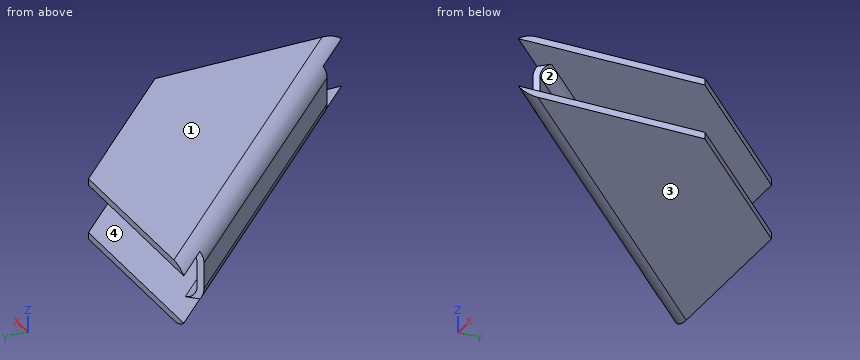
```python
from build123d import *

# Parameters (mm, degrees)
BOSS_EXTRUDE1_START = 6.35
BOSS_EXTRUDE1_DEPTH = 0.762
BOSS_EXTRUDE2_DEPTH = 12.7
FILLET1_R           = 2.54
FILLET2_R           = 4.064


with BuildPart() as part:
    # Sketch4 → Boss-Extrude1 (new, symmetric)
    with BuildSketch(Plane.XY.offset(BOSS_EXTRUDE1_START)):
        Polygon((86.76732538935741, 78.2227633784087), (131.2173253893574, 78.2227633784087), (162.78478969827367, 46.65529906949232), (162.78478969827367, 2.205299069492165), align=None)
    boss_extrude1 = extrude(amount=BOSS_EXTRUDE1_DEPTH, both=True)

    # Sketch5 → Boss-Extrude2 (add)
    with BuildSketch(Plane(origin=(0, 0, 5.588), x_dir=(-1, 0, 0), z_dir=(0, 0, -1))):
        Polygon((-153.41145680361603, 11.578631964150068), (-95.03979201666652, 69.95029675109956), (-96.11742275119471, 71.02792748562776), (-154.48908753814433, 12.656262698678363), align=None)
    extrude(amount=BOSS_EXTRUDE2_DEPTH)

    # Mirror2: Boss-Extrude1 across plane
    add(boss_extrude1.mirror(Plane.XY))

    # Fillet1
    fillet1_edges = [part.edges().sort_by_distance(p)[0] for p in [
        (125.30325514466952, 41.84209509215306, 5.588),
        (125.30325514466952, 41.84209509215306, -5.587999999999999),
    ]]
    fillet(fillet1_edges, radius=FILLET1_R)

    # Fillet2
    fillet2_edges = [part.edges().sort_by_distance(p)[0] for p in [
        (124.77605754381554, 40.21403122395043, 7.112),
        (124.77605754381554, 40.214031223950435, -7.112),
    ]]
    fillet(fillet2_edges, radius=FILLET2_R)


solid = part.part
```
Part model, mm, in its own coordinate system. Face numbers are marked on the shaded views. Round coordinates to 2 decimals unless told otherwise and drop trailing zeros. Write each loop counter-clockwise with the first axis right and the second up, starting at its lowest first coordinate (ties: lowest second). Pieces come first, ordered by that corner, then holes. Notation, with made-up numbers: M -19.75,72 L -5.75,72 A17 cw -5.75,97 Z; hole C 77,18.25 d8. An arc over 180 degrees is marked long. Answer as CSV lines item,"result". Start each with the question number.
1) Drop flat-ended pins along their axis: pin 1 (1 mm diameter, centred on y = 49, z = 3.5, fed in from +X); pin 2 (4 mm diameter, centred on x = 150, z = -2.5, fed in from -Y); pin 3 (2 mm diameter, centred on x = 112.5, z = -4.5, fed in from -Y). Give the stop position or say it passes through.
2) Drill centre lines: L1, parallel to Z at x = 105.5, y = 67; L2, parallel to X at y = 36, z = 2; L3, parallel to Y at x = 146.5, z = 6.25. Where is each one in solid material? Low to high.
3) Mould opens along Z. For the marked faces 1, 2, 3 and 4 say: +Z half, -Z half, draft (parallel to the pull), parting line (faces both ways), or undercut.
4) Band-saw the part on A-A (z = 1.5). List the corners of the cut face in (x, y).
Worked out:
1,pin 1,"x = 118.72"
1,pin 2,"y = 12.99"
1,pin 3,"y = 51.77"
2,L1,"-7.11 to -5.59, 5.59 to 7.11"
2,L2,"128.99 to 131.15"
2,L3,"20.7 to 62.94"
3,face 1,"+Z half"
3,face 2,"undercut"
3,face 3,"-Z half"
3,face 4,"undercut"
4,outline,"M 95.04,69.95 L 153.41,11.58 L 154.49,12.66 L 96.12,71.03 Z"
